Check sheet for the modelled part. Datum: model origin and axes. Units: mm. Face numbers are marked on the shaded views. A direction names the side the tool comes from. Round coordinates to 2 decimals unless told otherwise and drop trailing zeros. Write each loop counter-clockwise with the first axis right and the second up, starting at its lowest first coordinate (ties: lowest second). Pieces come first, ordered by that corner, then holes. Notation, with made-up numbers: (9.5, 62) -> (50.5, 62) arc R28 cw to (50.5, 93) -> close; hole circle Ø9 at (71, -27.75). An arc over 180 degrees is marked (long way). One line per item, written item: value. Start each with the question number.
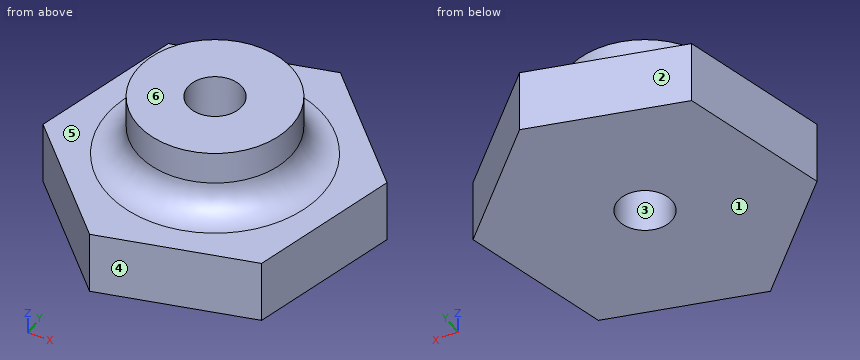
```python
from build123d import *

# Parameters (mm, degrees)
F0_R     = 3
F0_R_2   = 1.05
F1_DEPTH = 2.5
F2_DEPTH = 5
F3_R     = 1.2


with BuildPart() as f1:
    # F0 (on Top) → F1 (new body)
    with BuildSketch(Plane.XY):
        Polygon((1.545967, 5.797412), (-4.247722, 4.237553), (-5.79369, -1.559859), (-1.545967, -5.797412), (4.247722, -4.237553), (5.79369, 1.559859), align=None)
        Circle(F0_R, mode=Mode.SUBTRACT)
        Circle(F0_R)
        Circle(F0_R_2, mode=Mode.SUBTRACT)
    extrude(amount=F1_DEPTH)

    # F0 (on Top) → F2 (join)
    with BuildSketch(Plane.XY):
        Circle(F0_R)
        Circle(F0_R_2, mode=Mode.SUBTRACT)
    extrude(amount=F2_DEPTH)

    # F3
    f3_edges = [f1.edges().sort_by_distance(p)[0] for p in [
        (-3, 0, 2.5),
    ]]
    fillet(f3_edges, radius=F3_R)


solid = f1.part
```
1. Cross-section at A-A (z = 1.8). Record the cut outline in (x, y).
2. Material ranges on probe 1 along Y at (x, z) = (0, 4.7); probe 2 along Y at (x, z) = (0, 2.4); probe 3 along Z at (x, y) = (0, -4.5), recorded low to high.
3. Cross-section at D-D (z = 4.2). Record the cut outline in (x, y).
4. Release check for a two-part mould opening along Y. For the marked faces 1, 2, 3 and 4 record: +Y half, -Y half, draft (parallel to the pull), parting line (faces both ways), or undercut.
5. Depth check by flat-ended pin: pin 1 Ø1.5 at (x, z) = (-1, 1.5) entering from +Y; pin 2 Ø1.5 at (x, y) = (4, -1) entering from +Z; pin 3 Ø1.5 at (x, y) = (-4.5, -3.5) entering from +Z. Enter the tip coordinate at first touch or a pass-through.
6. Cross-section at B-B (y = 0). Record the cut outline in (x, z), plus the area to 3 significant figures.
7. Access from +Z, -Z, +X, -X, +Y, -Y to the whole of each face (thin tool, end or side, straight path). Record for the marked faces 5 and 6.
Working result:
1. outline: (-5.79, -1.56) -> (-1.55, -5.8) -> (4.25, -4.24) -> (5.79, 1.56) -> (1.55, 5.8) -> (-4.25, 4.24) -> close; hole circle Ø2.1 at (0, 0)
2. probe 1: y = -3 to -1.05, 1.05 to 3
2. probe 2: y = -5.38 to -1.05, 1.05 to 5.38
2. probe 3: z = 0 to 2.5
3. outline: circle Ø6 at (0, 0); hole circle Ø2.1 at (0, 0)
4. face 1: draft
4. face 2: +Y half
4. face 3: undercut
4. face 4: -Y half
5. pin 1: stops at y = 5.31
5. pin 2: stops at z = 2.83
5. pin 3: stops at z = 2.5
6. outline: (-5.38, 0) -> (-1.05, 0) -> (-1.05, 5) -> (-3, 5) -> (-3, 3.7) arc R1.2 cw to (-4.2, 2.5) -> (-5.38, 2.5) -> close; (1.05, 0) -> (5.38, 0) -> (5.38, 2.5) -> (4.2, 2.5) arc R1.2 cw to (3, 3.7) -> (3, 5) -> (1.05, 5) -> close
6. area: 32.0 mm^2
7. face 5: +Z
7. face 6: +Z, +X, -X, +Y, -Y
